Part model, mm, in its own coordinate system. A direction names the side the tool comes from. Round coordinates to 2 decimals unless told otherwise and drop trailing zeros. Write each loop counter-clockwise with the first axis right and the second up, starting at its lowest first coordinate (ties: lowest second). Pieces come first, ordered by that corner, then holes. Notation, with made-up numbers: (-8, 73) -> (18, 73) arc R14 cw to (18, 97) -> close; hole circle Ø2 at (-5.5, 7). An arc over 180 degrees is marked (long way). Return JSON: item names as keys, results as strings. Group by question number.
(1) Saw through at C-C (y = 12). List the corners of the cut face in (x, z), plus the area to 3 significant figures.
(2) Saw through at D-D (z = 14). List the corners of the cut face in (x, y).
(3) Drop flat-ended pins along their axis: pin 1 Ø14.5 at (x, y) = (14.5, 12) entering from +Z; pin 2 Ø4 at (x, z) = (38.5, 38.5) entering from +Y. Give the stop position or say it passes through.
(4) Saw through at A-A (z = 22.32). List the corners of the cut face in (x, y) (3 decimals).
(5) Mould opens along Z. For faces 1 (the cylindrical face through (28.45, -0.49, 37.46)), 2 (the flat face through (12.8, 0, 34.2)), 3 (the flat face through (24, 15, -1)) say: +Z half, -Z half, draft (parallel to the pull), parting line (faces both ways), or undercut.
(6) Saw through at B-B (x = 23.68). List the corners of the cut face in (y, z) (3 decimals).
(7) Drill centre lines: L1, parallel to X at y = -0.15, z = 22.32 (3 decimals); L2, parallel to Y at x = 43, z = 13. Where is each one in solid material? Low to high. Write a range as from..to.
(8) Tool access for faces 4 (the flat face through (47.36, -0.4, 23.3)), 5 (the flat face through (24, 16, 0)): list every direction of +Z, -Z, +X, -X, +Y, -Y with a clear straight run to the whole face (end or side of a thin tool).
from build123d import *

# Parameters (mm, degrees)
SKETCH10_W                   = 47.36
SKETCH10_H                   = 47.36
BASE_FLANGE1_DEPTH           = 1
EDGE_FLANGE1_STRIP_W         = 6
EDGE_FLANGE1_STRIP_H         = 1
EDGE_FLANGE1_STRIP_CUT_DEPTH = 47.36
EDGE_FLANGE1_DEPTH           = 47.36
SKETCH20_R                   = 15.875
CUT_EXTRUDE1_DEPTH           = 74.388958298


# Sheet-metal steps are written as plain solids
with BuildPart() as part:
    # Sketch10 → Base-Flange1 (new body)
    with BuildSketch(Plane(origin=(0, 0, 0), x_dir=(1, 0, 0), z_dir=(0, 1, 0))):
        with Locations((23.68, -23.68)):
            Rectangle(SKETCH10_W, SKETCH10_H)
    extrude(amount=-BASE_FLANGE1_DEPTH)

    # Edge-Flange1 strip (across the edge) → Edge-Flange1 strip cut (cut)
    with BuildSketch(Plane.ZY.offset(-47.36)):
        with Locations((-2, -0.5)):
            Rectangle(EDGE_FLANGE1_STRIP_W, EDGE_FLANGE1_STRIP_H)
    extrude(amount=EDGE_FLANGE1_STRIP_CUT_DEPTH, mode=Mode.SUBTRACT)

    # Edge-Flange1 section (across the edge) → Edge-Flange1 (add)
    with BuildSketch(Plane.ZY.offset(-47.36)):
        with BuildLine():
            Line((-1, 1), (-1, 30))
            Line((-1, 30), (0, 30))
            Line((0, 30), (0, 1))
            ThreePointArc((0, 1), (0.292893219, 0.292893219), (1, 0))
            Line((1, 0), (1, -1))
            ThreePointArc((1, -1), (-0.414213562, -0.414213562), (-1, 1))
        make_face()
    extrude(amount=EDGE_FLANGE1_DEPTH)

    # Sketch20 → Cut-Extrude1 (cut, through all)
    with BuildSketch(Plane(origin=(0, 0, 0), x_dir=(1, 0, 0), z_dir=(0, 1, 0))):
        with Locations(Location((23.68, -22.32, 0), (0, 0, 270))):
            Circle(SKETCH20_R)
    extrude(amount=-CUT_EXTRUDE1_DEPTH, mode=Mode.SUBTRACT)


solid = part.part
Computed values:
{
 "1": {"outline": "(0, -1) -> (47.36, -1) -> (47.36, 0) -> (0, 0) -> close", "area": "47.4 mm2"},
 "2": {"outline": "(0, -1) -> (10.16, -1) -> (10.16, 0) -> (0, 0) -> close; (37.2, -1) -> (47.36, -1) -> (47.36, 0) -> (37.2, 0) -> close"},
 "3": {"pin 1": "z = 0", "pin 2": "y = 0"},
 "4": {"outline": "(0, -1) -> (7.805, -1) -> (7.805, 0) -> (0, 0) -> close; (39.555, -1) -> (47.36, -1) -> (47.36, 0) -> (39.555, 0) -> close"},
 "5": {"face 1": "undercut", "face 2": "draft", "face 3": "-Z half"},
 "6": {"outline": "(-1, 1) arc R2 ccw to (1, -1) -> (30, -1) -> (30, 0) -> (1, 0) arc R1 cw to (0, 1) -> (0, 6.445) -> (-1, 6.445) -> close; (-1, 38.195) -> (0, 38.195) -> (0, 47.36) -> (-1, 47.36) -> close"},
 "7": {"L1": "0..7.805, 39.555..47.36", "L2": "-1..0"},
 "8": {"face 4": "+Z, -Z, +X, +Y, -Y", "face 5": "+Z, +X, -X, +Y"}
}
